Verification items for the finished model (mm, model axes). Give positions to 0.01 mm unless a question says otherwise; leave off trailing zeros. Write each loop counter-clockwise with the first axis right and the second up, starting at its lowest first coordinate (ties: lowest second). Pieces come first, ordered by that corner, then holes. Notation, with made-up numbers: (46.25, 36.25) -> (100.25, 36.25) arc R19 ccw to (100.25, 41.25) -> close; hole circle Ø5 at (-2, -27). An arc over 180 degrees is marked (long way). Use one line per item in the form item = value. Start each with the question number.
(1) Scan lines: L1, parallel to Z at x = 0, y = -0.9; L2, parallel to X at y = 0.15, z = 65; L3, parallel to Z at x = -1.25, y = -1.05. Record each from-to range of solid material in increasing order.
(2) Section check A-A, the plane z = 7.5. Record the cut outline in (x, y), plus the area to 3 significant figures.
(3) Section check C-C, the plane z = 65. Record the cut outline in (x, y), plus the area to 3 significant figures.
(4) Release check for a two-part mould opening along Z. For faces 1 (the face through (11.5, 0, 39)), 2 (the face through (0, 0, 80)), 3 (the face through (-1.21, 0.021, 9.397)) record: pulls with the +Z half, pulls with the -Z half, needs draft (parallel to the pull), parting line crosses it, or undercut.
(5) Depth check by flat-ended pin: pin 1 Ø1.6 at (x, z) = (-7.52, 5.14) entering from -Y. Enter the tip coordinate at first touch or a pass-through.
(6) Section check B-B, the plane x = 0. Record the cut outline in (y, z).
from build123d import *

# Parameters (mm, degrees)
ESQUISSE1_W             = 23
ESQUISSE1_H             = 3
BOSS_EXTRU_1_DEPTH      = 80
ESQUISSE3_R             = 1
ENL_V_MAT_EXTRU_2_DEPTH = 10
ESQUISSE4_R             = 1
ENL_V_MAT_EXTRU_3_DEPTH = 10
ESQUISSE5_R             = 2.25
ENL_V_MAT_EXTRU_4_DEPTH = 81.877994535


with BuildPart() as part:
    # Esquisse1 → Boss.-Extru.1 (new body)
    with BuildSketch(Plane.XY):
        Rectangle(ESQUISSE1_W, ESQUISSE1_H)
    extrude(amount=BOSS_EXTRU_1_DEPTH)

    # Esquisse3 → Enlèv. mat.-Extru.2 (cut)
    with BuildSketch(Plane.XZ.offset(1.5)):
        with Locations((0, 65)):
            Circle(ESQUISSE3_R)
    extrude(amount=-ENL_V_MAT_EXTRU_2_DEPTH, mode=Mode.SUBTRACT)

    # Esquisse4 → Enlèv. mat.-Extru.3 (cut)
    with BuildSketch(Plane(origin=(0, -1.5, 0), x_dir=(-1, 0, 0), z_dir=(0, -1, 0))):
        with Locations(Location((-6.497330661, -5.144161138, 0), (0, 0, 180))):
            Circle(ESQUISSE4_R)
        with Locations(Location((7.524836603, -5.144161138, 0), (0, 0, 180))):
            Circle(ESQUISSE4_R)
    extrude(amount=-ENL_V_MAT_EXTRU_3_DEPTH, mode=Mode.SUBTRACT)

    # Esquisse5 → Enlèv. mat.-Extru.4 (cut, through all)
    with BuildSketch(Plane(origin=(0, 1.5, 0), x_dir=(1, 0, 0), z_dir=(0, 1, 0))):
        with Locations(Location((0, -7.5, 0), (0, 0, 180))):
            Circle(ESQUISSE5_R)
    extrude(amount=-ENL_V_MAT_EXTRU_4_DEPTH, mode=Mode.SUBTRACT)


solid = part.part
Completed:
q1.L1 = 0 to 5.25, 9.75 to 64, 66 to 80
q1.L2 = -11.5 to -1, 1 to 11.5
q1.L3 = 0 to 5.63, 9.37 to 80
q2.outline = (-11.5, -1.5) -> (-2.25, -1.5) -> (-2.25, 1.5) -> (-11.5, 1.5) -> close; (2.25, -1.5) -> (11.5, -1.5) -> (11.5, 1.5) -> (2.25, 1.5) -> close
q2.area = 55.5 mm²
q3.outline = (-11.5, -1.5) -> (-1, -1.5) -> (-1, 1.5) -> (-11.5, 1.5) -> close; (1, -1.5) -> (11.5, -1.5) -> (11.5, 1.5) -> (1, 1.5) -> close
q3.area = 63.0 mm²
q4.face_1 = needs draft
q4.face_2 = pulls with the +Z half
q4.face_3 = undercut
q5.pin_1 = through
q6.outline = (-1.5, 0) -> (1.5, 0) -> (1.5, 5.25) -> (-1.5, 5.25) -> close; (-1.5, 9.75) -> (1.5, 9.75) -> (1.5, 64) -> (-1.5, 64) -> close; (-1.5, 66) -> (1.5, 66) -> (1.5, 80) -> (-1.5, 80) -> close
